```python
from build123d import *

# Parameters (mm, degrees)
SKETCH1_W            = 130
SKETCH1_H            = 65
BOSS_EXTRUDE1_DEPTH  = 4
SKETCH4_R            = 3.5
SKETCH4_R_2          = 1.5
BOSS_EXTRUDE3_DEPTH  = 70
SKETCH5_2_W          = 6
SKETCH5_2_H          = 26
BOSS_EXTRUDE5_DEPTH  = 36
SKETCH5_W            = 6
SKETCH5_H            = 26
BOSS_EXTRUDE4_DEPTH  = 36
SKETCH7_R            = 1.5
CUT_EXTRUDE2_DEPTH   = 10
FILLET1_R            = 6
FILLET1_OF_MIRROR1_R = 6
SKETCH10_R           = 2
CUT_EXTRUDE3_DEPTH   = 10
FILLET2_R            = 3


with BuildPart() as part:
    # Sketch1 → Boss-Extrude1 (new body)
    with BuildSketch(Plane(origin=(0, 0, 0), x_dir=(1, 0, 0), z_dir=(0, 1, 0))):
        Rectangle(SKETCH1_W, SKETCH1_H)
    extrude(amount=-BOSS_EXTRUDE1_DEPTH)

    # Sketch4 → Boss-Extrude3 (add)
    # profile 1 of 4: a face of its own
    with BuildSketch(Plane(origin=(0, 0, 0), x_dir=(1, 0, 0), z_dir=(0, 1, 0))):
        with Locations(Location((-58, 25.5, 0), (0, 0, 270))):
            Circle(SKETCH4_R)
        with Locations(Location((-58, 25.5, 0), (0, 0, 270))):
            Circle(SKETCH4_R_2, mode=Mode.SUBTRACT)
    # profile 2 of 4: a face of its own
    with BuildSketch(Plane(origin=(0, 0, 0), x_dir=(1, 0, 0), z_dir=(0, 1, 0))):
        with Locations(Location((58, 25.5, 0), (0, 0, 270))):
            Circle(SKETCH4_R)
        with Locations(Location((58, 25.5, 0), (0, 0, 270))):
            Circle(SKETCH4_R_2, mode=Mode.SUBTRACT)
    # profile 3 of 4: a face of its own
    with BuildSketch(Plane(origin=(0, 0, 0), x_dir=(1, 0, 0), z_dir=(0, 1, 0))):
        with Locations(Location((-58, -25.5, 0), (0, 0, 270))):
            Circle(SKETCH4_R)
        with Locations(Location((-58, -25.5, 0), (0, 0, 270))):
            Circle(SKETCH4_R_2, mode=Mode.SUBTRACT)
    # profile 4 of 4: a face of its own
    with BuildSketch(Plane(origin=(0, 0, 0), x_dir=(1, 0, 0), z_dir=(0, 1, 0))):
        with Locations(Location((58, -25.5, 0), (0, 0, 270))):
            Circle(SKETCH4_R)
        with Locations(Location((58, -25.5, 0), (0, 0, 270))):
            Circle(SKETCH4_R_2, mode=Mode.SUBTRACT)
    extrude(amount=BOSS_EXTRUDE3_DEPTH)

    # Sketch5<2> → Boss-Extrude5 (add)
    with BuildSketch(Plane(origin=(0, 0, 0), x_dir=(1, 0, 0), z_dir=(0, 1, 0))):
        with Locations((62, 0)):
            Rectangle(SKETCH5_2_W, SKETCH5_2_H)
    boss_extrude5 = extrude(amount=BOSS_EXTRUDE5_DEPTH)

    # Sketch5 → Boss-Extrude4 (add)
    with BuildSketch(Plane(origin=(0, 0, 0), x_dir=(1, 0, 0), z_dir=(0, 1, 0))):
        with Locations((62, 0)):
            Rectangle(SKETCH5_W, SKETCH5_H)
    extrude(amount=BOSS_EXTRUDE4_DEPTH)

    # Sketch7 → Cut-Extrude2 (cut)
    with BuildSketch(Plane(origin=(65, 0, 0), x_dir=(0, 0, -1), z_dir=(1, 0, 0))):
        with Locations((-9, 32)):
            Circle(SKETCH7_R)
        with Locations((9, 32)):
            Circle(SKETCH7_R)
    cut_extrude2 = extrude(amount=-CUT_EXTRUDE2_DEPTH, mode=Mode.SUBTRACT)

    # Fillet1
    fillet1_edges = [part.edges().sort_by_distance(p)[0] for p in [
        (62, 0, -13),
        (59, 0, 0),
        (62, 0, 13),
        (62, 36, -13),
        (62, 36, 13),
    ]]
    fillet(fillet1_edges, radius=FILLET1_R)

    # Mirror1: Boss-Extrude5, Cut-Extrude2 across plane
    add(boss_extrude5.mirror(Plane(origin=(0, 0, 0), x_dir=(0, 0, 1), z_dir=(1, 0, 0))))
    add(cut_extrude2.mirror(Plane(origin=(0, 0, 0), x_dir=(0, 0, 1), z_dir=(1, 0, 0))), mode=Mode.SUBTRACT)

    # Fillet1 of Mirror1
    fillet1_of_mirror1_edges = [part.edges().sort_by_distance(p)[0] for p in [
        (-62, 0, -13),
        (-59, 0, 0),
        (-62, 0, 13),
        (-62, 36, -13),
        (-62, 36, 13),
    ]]
    fillet(fillet1_of_mirror1_edges, radius=FILLET1_OF_MIRROR1_R)

    # Sketch10 → Cut-Extrude3 (cut)
    with BuildSketch(Plane(origin=(0, 0, 0), x_dir=(1, 0, 0), z_dir=(0, 1, 0))):
        with Locations(Location((0, 22, 0), (0, 0, 270))):
            Circle(SKETCH10_R)
        with Locations(Location((0, -22, 0), (0, 0, 270))):
            Circle(SKETCH10_R)
    extrude(amount=-CUT_EXTRUDE3_DEPTH, mode=Mode.SUBTRACT)

    # Fillet2
    fillet2_edges = [part.edges().sort_by_distance(p)[0] for p in [
        (-58, 0, -29),
        (58, 0, -29),
        (-58, 0, 22),
        (58, 0, 22),
    ]]
    fillet(fillet2_edges, radius=FILLET2_R - 0.0001)  # a hair under: the kernel refuses the full size


solid = part.part
```
Check sheet for the modelled part. Datum: model origin and axes. Units: mm. A direction names the side the tool comes from. Round coordinates to 2 decimals unless told otherwise and drop trailing zeros. Loops run counter-clockwise (first coordinate to the right, second up) from the corner with the lowest first, then second, coordinate; pieces in that order, holes last. Notation, with made-up numbers: (57, -22) -> (94, -22) arc R26 ccw to (94, 3) -> close; hole circle Ø10 at (29, -19.5). An arc over 180 degrees is marked (long way). Answer in a Markdown table with one row per item.
Q1. Release check for a two-part mould opening along X. For faces 4 (the face through (62, 18, -13)), 5 (the face through (-61.105, 36.031, 27.115)) record: released by +X, released by -X, zero draft, split by the parting line, or undercut.
Data:
| item | result |
|---|---|
| face 4 | zero draft |
| face 5 | undercut |
Q2. Sectioned sample at C-C on z = -25.5. Enter the section's corners in (x, y).
Data:
| item | result |
|---|---|
| outline | (-65, -4) -> (65, -4) -> (65, 0) -> (64.5, 0) arc R3 cw to (61.5, 3) -> (61.5, 70) -> (59.5, 70) -> (59.5, 0) -> (56.5, 0) -> (56.5, 70) -> (54.5, 70) -> (54.5, 3) arc R3 cw to (51.5, 0) -> (-51.5, 0) arc R3 cw to (-54.5, 3) -> (-54.5, 70) -> (-56.5, 70) -> (-56.5, 0) -> (-59.5, 0) -> (-59.5, 70) -> (-61.5, 70) -> (-61.5, 3) arc R3 cw to (-64.5, 0) -> (-65, 0) -> close |
Q3. Sectioned sample at A-A on y = 38.5. Enter the section's corners in (x, z).
Data:
| item | result |
|---|---|
| outline | circle Ø7 at (-58, -25.5); circle Ø7 at (-58, 25.5); circle Ø7 at (58, -25.5); circle Ø7 at (58, 25.5); hole circle Ø3 at (-58, -25.5); hole circle Ø3 at (-58, 25.5); hole circle Ø3 at (58, -25.5); hole circle Ø3 at (58, 25.5) |
Q4. Thickness scan on L1, parallel to X at y = 49, z = 25.5; L2, parallel to X at y = 10, z = 4; L3, parallel to X at y = 29, z = -25. Record the ranges inside material, lowest first.
Data:
| item | result |
|---|---|
| L1 | x = -61.5 to -59.5, -56.5 to -54.5, 54.5 to 56.5, 59.5 to 61.5 |
| L2 | x = -65 to -59, 59 to 65 |
| L3 | x = -61.46 to -59.41, -56.59 to -54.54, 54.54 to 56.59, 59.41 to 61.46 |
Q5. Go/stop test with flat-tipped pins: P1, Ø5, axis at x = 60.5, z = 0.5, coming from the +Y side; P2, Ø5, axis at x = 63, y = 19.5, coming from the +Z side; P3, Ø6.5, axis at x = 0, z = -22, coming from the +Y side. Record where each tip stops, or that it passes through.
Data:
| item | result |
|---|---|
| P1 | stops at y = 36 |
| P2 | stops at z = 27.95 |
| P3 | stops at y = 0 |
Q6. Set-up check for faces 1 (the face through (-62.042, 34.196, -11.289)), 2 (the face through (-60, 70, 25)), 3 (the face through (-58, 0, -26)): record each of +Z, -Z, +X, -X, +Y, -Y from which the full face is reachable in a straight line by a thin tool's end or side.
Data:
| item | result |
|---|---|
| face 1 | +X, -X, +Y |
| face 2 | +Z, -Z, +X, -X, +Y |
| face 3 | +Y |
Q7. Sectioned sample at B-B on x = 0. Enter the section's corners in (y, z), then the cut area to 3 significant figures.
Data:
| item | result |
|---|---|
| outline | (-4, -32.5) -> (0, -32.5) -> (0, -24) -> (-4, -24) -> close; (-4, -20) -> (0, -20) -> (0, 20) -> (-4, 20) -> close; (-4, 24) -> (0, 24) -> (0, 32.5) -> (-4, 32.5) -> close |
| area | 228 mm^2 |
Q8. Sectioned sample at D-D on x = 15.5. Enter the section's corners in (y, z), then the cut area to 3 significant figures.
Data:
| item | result |
|---|---|
| outline | (-4, -32.5) -> (0, -32.5) -> (0, 32.5) -> (-4, 32.5) -> close |
| area | 260 mm^2 |
